Geometry check sheet. Reference: the model listing, model coordinates, mm. Face numbers are marked on the shaded views. A direction names the side the tool comes from. Give positions to 0.01 mm unless a question says otherwise; leave off trailing zeros. Order: outer loops, then holes, each group sorted by start corner. A loop starts at its lowest first (then second) coordinate and runs counter-clockwise, first axis right, second up. Notation, with made-up numbers: M 39.25,47.5 L 45.25,47.5 A11 ccw 45.25,53.5 Z; hole C 61,21.5 d11. An arc over 180 degrees is marked long. One line per question, with ' | ' between items. Start each with the question number.
from build123d import *

# Parameters (mm, degrees)
BOSS_EXTRUDE1_DEPTH = 15
FILLET2_R           = 10
SKETCH8_R           = 1.6
CUT_EXTRUDE6_DEPTH  = 29.681007074
CUT_EXTRUDE7_REACH  = 30.681
SKETCH9_W           = 7.5
SKETCH9_H           = 10
CUT_EXTRUDE8_REACH  = 30.681
SKETCH10_R          = 1.6
FILLET3_R           = 2
FILLET6_R           = 2
SKETCH11_R          = 2.05
CUT_EXTRUDE9_DEPTH  = 10
SKETCH12_R          = 2.25
CUT_EXTRUDE10_DEPTH = 14.5


with BuildPart() as part:
    # Sketch2 → Boss-Extrude1 (new body)
    with BuildSketch(Plane.XY):
        with BuildLine():
            Line((-2.5, -6.008335649), (-2.5, -21.008335649))
            Line((-2.5, -21.008335649), (-5, -21.008335649))
            Line((-5, -21.008335649), (-5, -6.008335649))
            Line((-5, -6.008335649), (-5, -5.590169944))
            ThreePointArc((-5, -5.590169944), (0, 7.5), (5, -5.590169944))
            Line((5, -5.590169944), (5, -6.008335649))
            Line((5, -6.008335649), (5, -21.008335649))
            Line((5, -21.008335649), (2.5, -21.008335649))
            Line((2.5, -21.008335649), (2.5, -6.008335649))
            Line((2.5, -6.008335649), (-2.5, -6.008335649))
        make_face()
    extrude(amount=BOSS_EXTRUDE1_DEPTH)

    # Fillet2
    fillet2_edges = [part.edges().sort_by_distance(p)[0] for p in [
        (-5, -5.590169944, 7.5),
        (5, -5.590169944, 7.5),
    ]]
    fillet(fillet2_edges, radius=FILLET2_R)

    # Sketch8 → Cut-Extrude6 (cut, through all)
    with BuildSketch(Plane(origin=(5, 0, 0), x_dir=(0, 0, -1), z_dir=(1, 0, 0))):
        with Locations((-3.5, -16.008335649)):
            Circle(SKETCH8_R)
    extrude(amount=-CUT_EXTRUDE6_DEPTH, mode=Mode.SUBTRACT)

    # Sketch9 → Cut-Extrude7 (cut, up to next)
    with BuildSketch(Plane.ZY.offset(5), mode=Mode.PRIVATE) as cut_extrude7_sk1:
        with Locations((11.25, -16.008335649)):
            Rectangle(SKETCH9_W, SKETCH9_H)
    cut_extrude7_tool1 = extrude(cut_extrude7_sk1.sketch, amount=-CUT_EXTRUDE7_REACH, mode=Mode.PRIVATE) & part.part
    add(cut_extrude7_tool1.solids().sort_by_distance((-5, -16.008336, 11.25))[0], mode=Mode.SUBTRACT)

    # Sketch10 → Cut-Extrude8 (cut, up to next)
    with BuildSketch(Plane(origin=(5, 0, 0), x_dir=(0, 0, -1), z_dir=(1, 0, 0)), mode=Mode.PRIVATE) as cut_extrude8_sk1:
        with Locations((-11.5, -16.008335649)):
            Circle(SKETCH10_R)
    cut_extrude8_tool1 = extrude(cut_extrude8_sk1.sketch, amount=-CUT_EXTRUDE8_REACH, mode=Mode.PRIVATE) & part.part
    add(cut_extrude8_tool1.solids().sort_by_distance((5, -16.008336, 11.5))[0], mode=Mode.SUBTRACT)

    # Fillet3
    fillet3_edges = [part.edges().sort_by_distance(p)[0] for p in [
        (-2.5, -6.008335649, 7.5),
        (2.5, -21.008335649, 7.5),
        (2.5, -6.008335649, 7.5),
        (-2.5, -21.008335649, 3.75),
    ]]
    fillet(fillet3_edges, radius=FILLET3_R)

    # Fillet6
    fillet6_edges = [part.edges().sort_by_distance(p)[0] for p in [
        (-3.75, -11.008335649, 15),
        (-3.75, -11.008335649, 7.5),
    ]]
    fillet(fillet6_edges, radius=FILLET6_R)

    # Sketch11 → Cut-Extrude9 (cut)
    with BuildSketch(Plane(origin=(0, 0, 0), x_dir=(-1, 0, 0), z_dir=(0, 0, -1))):
        Circle(SKETCH11_R)
    extrude(amount=-CUT_EXTRUDE9_DEPTH, mode=Mode.SUBTRACT)

    # Sketch12 → Cut-Extrude10 (cut, symmetric)
    with BuildSketch(Plane(origin=(5, 0, 0), x_dir=(0, 0, -1), z_dir=(1, 0, 0))):
        with Locations((-7.6, 0)):
            Circle(SKETCH12_R)
    extrude(amount=CUT_EXTRUDE10_DEPTH, both=True, mode=Mode.SUBTRACT)


solid = part.part
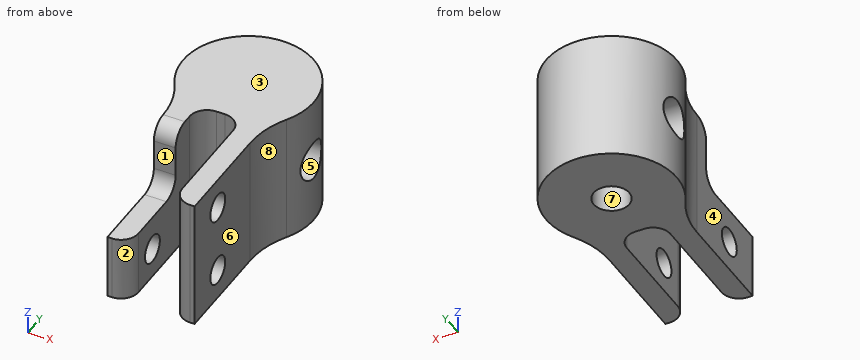
Item 1: Cross-section at D-D, the plane z = 11.5. Record the cut outline in (x, y).
Item 2: Cross-section at B-B, the plane y = 0. Record the cut outline in (x, z), plus the area to 3 significant figures.
Item 3: Cross-section at A-A, the plane z = 3.5. Record the cut outline in (x, y).
Item 4: Set-up check for the marked faces 1, 2, 3, 4 and 5: record each of +Z, -Z, +X, -X, +Y, -Y from which the full face is reachable in a straight line by a thin tool's end or side.
Item 5: Material ranges on line 1 along X through (y, z) = (-14, 3); line 2 along X through (y, z) = (0, 3.5); line 3 along X through (y, z) = (-15.5, 13.25), recorded low to high.
Item 6: Mould release check, pull along Y, two halves, no side actions. Record for the marked faces 6, 7 and 8: released by +Y, released by -Y, zero draft, split by the parting line, or undercut.
Item 7: Cross-section at C-C, the plane x = 0. Record the cut outline in (y, z), plus the area to 3 significant figures.
Item 8: Depth check by flat-ended pin: pin 1 (1.2 mm diameter, centred on x = -4, z = 12, fed in from -Y); pin 2 (3.5 mm diameter, centred on y = -16.01, z = 3.5, fed in from +X); pin 3 (6 mm diameter, centred on x = 0, z = 8, fed in from -Y); pin 4 (4 mm diameter, centred on y = 0, z = 7.6, fed in from +X). Enter the tip coordinate at first touch or a pass-through.
Outcome:
1) outline: M -6.43,-3.86 A10 cw -5,-9.01 L -5,-11.01 L -2.5,-11.01 L -2.5,-8.01 A2 cw -0.5,-6.01 L 0.5,-6.01 A2 cw 2.5,-8.01 L 2.5,-14.41 L 5,-14.41 L 5,-9.01 A10 cw 6.43,-3.86 A7.5 ccw long Z; M 2.5,-19.01 A2 ccw 4.5,-21.01 L 5,-21.01 L 5,-17.61 L 2.5,-17.61 Z
2) outline: M -7.5,0 L -2.05,0 L -2.05,5.35 L -7.5,5.35 Z; M -7.5,9.85 L -2.05,9.85 L -2.05,10 L 2.05,10 L 2.05,9.85 L 7.5,9.85 L 7.5,15 L -7.5,15 Z; M 2.05,0 L 7.5,0 L 7.5,5.35 L 2.05,5.35 Z | area: 135 mm²
3) outline: M -6.43,-3.86 A10 cw -5,-9.01 L -5,-14.41 L -2.5,-14.41 L -2.5,-8.01 A2 cw -0.5,-6.01 L 0.5,-6.01 A2 cw 2.5,-8.01 L 2.5,-14.41 L 5,-14.41 L 5,-9.01 A10 cw 6.43,-3.86 A7.5 ccw long Z; M -5,-21.01 L -4.5,-21.01 A2 ccw -2.5,-19.01 L -2.5,-17.61 L -5,-17.61 Z; M 2.5,-19.01 A2 ccw 4.5,-21.01 L 5,-21.01 L 5,-17.61 L 2.5,-17.61 Z; hole C 0,0 d4.1
4) face 1: +Z, -X, -Y | face 2: +Z, -Z, -Y | face 3: +Z, +X, -X, +Y, -Y | face 4: +Z, -Z, -X, -Y | face 5: +X, -X
5) line 1: x = -5 to -2.5, 2.5 to 5 | line 2: x = -7.5 to -2.05, 2.05 to 7.5 | line 3: x = 2.5 to 5
6) face 6: zero draft | face 7: undercut | face 8: released by -Y
7) outline: M -6.01,0 L -2.05,0 L -2.05,6.67 A2.25 cw -2.05,8.53 L -2.05,10 L 2.05,10 L 2.05,8.53 A2.25 cw 2.05,6.67 L 2.05,0 L 7.5,0 L 7.5,15 L -6.01,15 Z | area: 161 mm²
8) pin 1: stops at y = -11.01 | pin 2: stops at x = 5 | pin 3: stops at y = -20.33 | pin 4: passes through
